For this review, use the dimensioned drawing (mm, ordinates from the lowest corner) and the shaded views. A direction names the side the tool comes from. Give positions to 0.01 mm unless a question says otherwise; leave off trailing zeros. Order: outer loops, then holes, each group sorted by start corner. A loop starts at its lowest first (then second) coordinate and runs counter-clockwise, first axis right, second up. Notation, with made-up numbers: (44.25, 10) - (73.25, 10) arc R18 cw to (73.25, 15) - close; hole circle Ø6 at (81, -12). An arc over 180 degrees is marked (long way). Use a Markdown table: item, result. Add a question column.
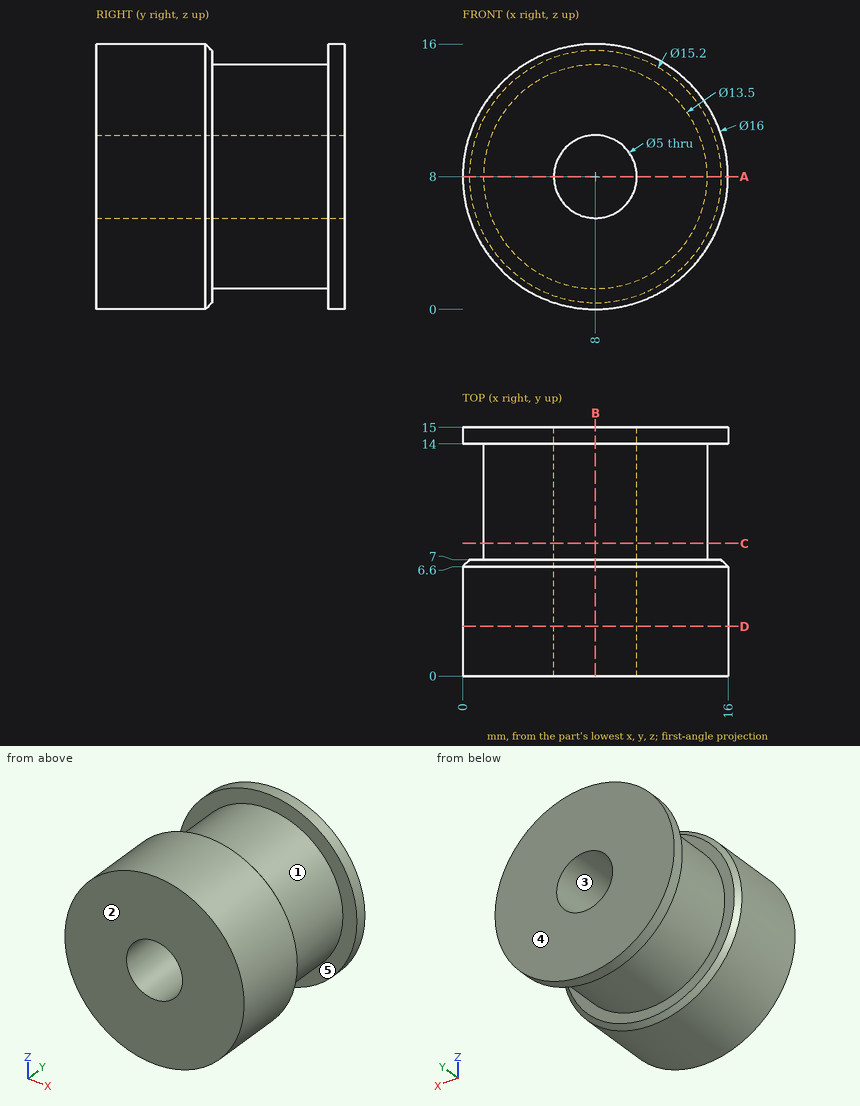
Q1. We need section A-A (z = 8). Write out the cut boundary in (x, y), plus the area to 3 significant figures.
Q2. We need section D-D (y = 3). Write out the cut boundary in (x, z), plus the area to 3 significant figures.
Q3. Wall thickness on probe 1 along Z at (x, y) = (8, 6.5); probe 2 along Z at (x, y) = (8, 9.5); probe 3 along X at (y, z) = (8.5, 2.75): over which ranges is each line inside the solid? List them lowest first.
Q4. Draft analysis for pull direction Y (two halves, no side actions). For the marked faces 3, 4 and 5, state which applies: pulls with the +Y half, pulls with the -Y half, needs draft (parallel to the pull), parting line crosses it, or undercut.
Q5. We need section B-B (x = 8). Write out the cut boundary in (y, z), plus the area to 3 significant figures.
Q6. We need section C-C (y = 8). Write out the cut boundary in (x, z).
Q7. Machinability: for the marked faces 1 and 2, which of the approach directions +Z, -Z, +X, -X, +Y, -Y give a long, thin tool a straight path to every point of the face, cutting with its end or side? Answer none if there is none.
Q8. Clearance check with flat-ended pins moving along their axes: P1, Ø5, axis at y = 12, z = 14, coming from the +X side; P2, Ø1, axis at y = 10, z = 3.5, coming from the -X side; P3, Ø6, axis at x = 13.5, y = 10, coming from the +Z side. State where each tip first meets the part, or that it passes through.
Here are the results:
| question | item | result |
|---|---|---|
| 1 | outline | (0, 0) - (5.5, 0) - (5.5, 15) - (0, 15) - (0, 14) - (1.25, 14) - (1.25, 7) - (0.4, 7) - (0, 6.6) - close; (10.5, 0) - (16, 0) - (16, 6.6) - (15.6, 7) - (14.75, 7) - (14.75, 14) - (16, 14) - (16, 15) - (10.5, 15) - close |
| 1 | area | 147 mm2 |
| 2 | outline | circle Ø16 at (8, 8); hole circle Ø5 at (8, 8) |
| 2 | area | 181 mm2 |
| 3 | probe 1 | 0 to 5.5, 10.5 to 16 |
| 3 | probe 2 | 1.25 to 5.5, 10.5 to 14.75 |
| 3 | probe 3 | 3.76 to 12.24 |
| 4 | face 3 | needs draft |
| 4 | face 4 | pulls with the +Y half |
| 4 | face 5 | undercut |
| 5 | outline | (0, 0) - (6.6, 0) - (7, 0.4) - (7, 1.25) - (14, 1.25) - (14, 0) - (15, 0) - (15, 5.5) - (0, 5.5) - close; (0, 10.5) - (15, 10.5) - (15, 16) - (14, 16) - (14, 14.75) - (7, 14.75) - (7, 15.6) - (6.6, 16) - (0, 16) - close |
| 5 | area | 147 mm2 |
| 6 | outline | circle Ø13.5 at (8, 8); hole circle Ø5 at (8, 8) |
| 7 | face 1 | none |
| 7 | face 2 | +Z, -Z, +X, -X, -Y |
| 8 | P1 | x = 14.61 |
| 8 | P2 | x = 2.56 |
| 8 | P3 | z = 14.27 |
